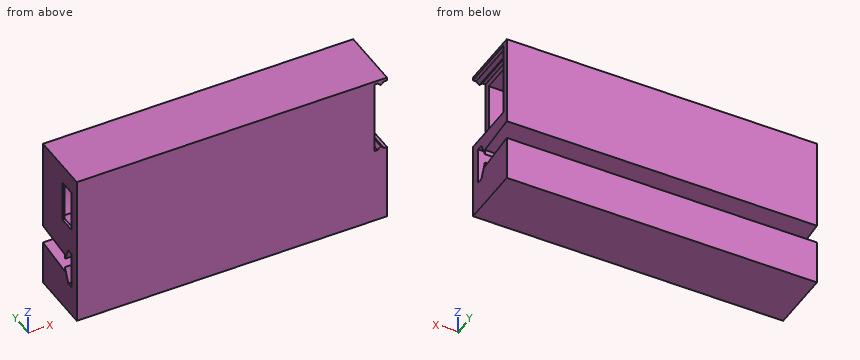
```python
from build123d import *

# Parameters (mm, degrees)
P_IDAT_VYSUNUT_M2_DEPTH  = 100
ODEBRAT_START            = -1.2
SKICA3_W                 = 20
SKICA3_H                 = 12
ODEBRAT_VYSUNUT_M1_DEPTH = 98
SKICA4_W                 = 13.4
SKICA4_H                 = 5.6
ODEBRAT_VYSUNUT_M2_DEPTH = 95
SKICA5_W                 = 2
SKICA5_H                 = 2
ODEBRAT_VYSUNUT_M3_DEPTH = 9
ODEBRAT_VYSUNUT_M6_DEPTH = 98
ODEBRAT_VYSUNUT_M8_DEPTH = 18


with BuildPart() as part:
    # Skica2 → Přidat vysunutím2 (new body)
    with BuildSketch(Plane(origin=(0, 0, 0), x_dir=(0, 0, -1), z_dir=(1, 0, 0))):
        Polygon((4.558367755, 10), (-25, 10), (-25, -10), (25, -10), (25, 10), (10.59358807, 10), (12, -2.961048892), (10.5, -2.961048892), (15, -5), (15, -7), (3, -7), (3, -5), (7.5, -2.961048892), (5.964779685, -2.961048892), align=None)
    extrude(amount=P_IDAT_VYSUNUT_M2_DEPTH)

    # Skica3 → Odebrat vysunutím1 (cut)
    with BuildSketch(Plane(origin=(100, 0, 0), x_dir=(0, 0, -1), z_dir=(1, 0, 0)).offset(ODEBRAT_START)):
        with Locations((-12, -2)):
            Rectangle(SKICA3_W, SKICA3_H)
    extrude(amount=-ODEBRAT_VYSUNUT_M1_DEPTH, mode=Mode.SUBTRACT)

    # Skica4 → Odebrat vysunutím2 (cut)
    with BuildSketch(Plane.ZY):
        with Locations((12.3, -4.2)):
            Rectangle(SKICA4_W, SKICA4_H)
    extrude(amount=-ODEBRAT_VYSUNUT_M2_DEPTH, mode=Mode.SUBTRACT)

    # Skica5 → Odebrat vysunutím3 (cut)
    with BuildSketch(Plane(origin=(0, 0, -3), x_dir=(-1, 0, 0), z_dir=(0, 0, -1))):
        with Locations((-94, -6)):
            Rectangle(SKICA5_W, SKICA5_H)
    extrude(amount=-ODEBRAT_VYSUNUT_M3_DEPTH, mode=Mode.SUBTRACT)

    # Skica10 → Odebrat vysunutím6 (cut)
    with BuildSketch(Plane(origin=(100, 0, 0), x_dir=(0, 0, -1), z_dir=(1, 0, 0)).offset(ODEBRAT_START)):
        with BuildLine():
            Line((-22, 4), (-2, 4))
            ThreePointArc((-2, 4), (-12, 7.510004003), (-22, 4))
        make_face()
    extrude(amount=-ODEBRAT_VYSUNUT_M6_DEPTH, mode=Mode.SUBTRACT)

    # Skica17 → Odebrat vysunutím8 (cut)
    with BuildSketch(Plane.XZ.offset(10)):
        Polygon((98, 12), (96, 12), (96, 0), (97, 0), (98, 1), align=None)
        Polygon((100, 0), (98, 12), (98, 1), (99, 0), align=None)
        Polygon((100, 12), (98, 12), (100, 0), align=None)
        Polygon((98, 23), (98, 12), (100, 12), (100, 24), (99, 24), align=None)
        Polygon((98, 12), (96, 24), (96, 12), align=None)
        Polygon((97, 24), (96, 24), (98, 12), (98, 23), align=None)
    extrude(amount=-ODEBRAT_VYSUNUT_M8_DEPTH, mode=Mode.SUBTRACT)


solid = part.part
```
The listing builds one solid part. Answer for the finished solid, in the listing's coordinates (mm). Coordinates: 2 decimals unless noted, no trailing zeros. Loops run counter-clockwise (first coordinate to the right, second up) from the corner with the lowest first, then second, coordinate; pieces in that order, holes last. Notation, with made-up numbers: (-25.75, -23) - (22.25, -23) arc R16 cw to (22.25, -8) - close; hole circle Ø2 at (64.25, 45.25). An arc over 180 degrees is marked (long way). Use a Markdown table: item, result. Add a question column.
1) The part is cut by section A-A, the plane x = 87. Give the vertices of the cut face in (y, z).
2) The part is cut by section B-B, the plane z = 15. Give the vertices of the cut face in (x, y), and give its area (3 significant figures).
3) Given pin 1 (8 mm diameter, centred on y = -3.5, z = 7.5, fed in from +X); pin 2 (0.6 mm diameter, centred on y = -6, z = 0.5, fed in from +X); pin 3 (2 mm diameter, centred on x = 97.5, z = 15, fed in from -Y), each flat-ended and moving along its own axis, determine where each tip first touches the part or whether it passes through.
4) The part is cut by section C-C, the plane y = 1.75. Give the vertices of the cut face in (x, z).
5) Find the intervals of material crossed by line 1 (Z direction, x = 87, y = -6.25); line 2 (Z direction, x = 24.5, y = 2.75); line 3 (X direction, y = 4.75, z = 4.5), in increasing order.
Here are the results:
| question | item | result |
|---|---|---|
| 1 | outline | (-10, -25) - (10, -25) - (10, -10.59) - (-2.96, -12) - (-2.96, -10.5) - (-5, -15) - (-7, -15) - (-7, -3) - (-5, -3) - (-2.96, -7.5) - (-2.96, -5.96) - (10, -4.56) - (10, 25) - (-10, 25) - close; hole (-8, 2) - (4, 2) arc R16 ccw to (4, 22) - (-8, 22) - close |
| 2 | outline | (0, -10) - (96, -10) - (96, -8) - (0.8, -8) - (0.8, -7) - (0, -7) - close; (0, -1.4) - (0.8, -1.4) - (0.8, 7.23) - (96, 7.23) - (96, 8) - (100, 8) - (100, 10) - (0, 10) - close |
| 2 | area | 474 mm^2 |
| 3 | pin 1 | stops at x = 0.8 |
| 3 | pin 2 | stops at x = 98.8 |
| 3 | pin 3 | stops at y = 8 |
| 4 | outline | (0, -25) - (100, -25) - (100, -11.49) - (0, -11.49) - close; (0, -5.45) - (100, -5.45) - (100, 0) - (99, 0) - (98, 1) - (97, 0) - (96, 0) - (96, 2) - (0.8, 2) - (0.8, 22) - (96, 22) - (96, 24) - (97, 24) - (98, 23) - (99, 24) - (100, 24) - (100, 25) - (0, 25) - close |
| 5 | line 1 | z = -25 to -15, -3 to 2, 22 to 25 |
| 5 | line 2 | z = -25 to -11.38, -5.35 to 2, 22 to 25 |
| 5 | line 3 | x = 0 to 0.8 |
